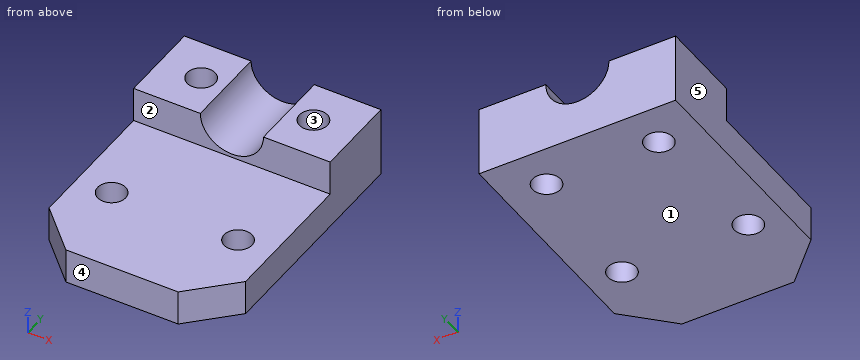
from build123d import *

# Parameters (mm, degrees)
SKETCH_1_R          = 2
EXTRUDE_1_DEPTH     = 10
CUT_EXTRUDE_2_REACH = 1024.045
SKETCH_2_W          = 6.505809731
SKETCH_2_H          = 33.357060804
SKETCH_3_R          = 4.5
CUT_EXTRUDE_3_DEPTH = 20


with BuildPart() as part:
    # 草图1 → 拉伸1 (new body)
    with BuildSketch(Plane.XY):
        Polygon((1243.510947309, 989.612625701), (1243.510947309, 1021.612625701), (1271.510947309, 1021.612625701), (1271.510947309, 989.612625701), (1265.510947309, 983.612625701), (1249.510947309, 983.612625701), align=None)
        with Locations((1265.510947309, 1015.612625701)):
            Circle(SKETCH_1_R, mode=Mode.SUBTRACT)
        with Locations((1249.510947309, 1015.612625701)):
            Circle(SKETCH_1_R, mode=Mode.SUBTRACT)
        with Locations((1248.510947309, 996.112625701)):
            Circle(SKETCH_1_R, mode=Mode.SUBTRACT)
        with Locations((1266.510947309, 996.112625701)):
            Circle(SKETCH_1_R, mode=Mode.SUBTRACT)
    extrude(amount=EXTRUDE_1_DEPTH)

    # 草图2 → 拉伸2 (cut, up to next)
    with BuildSketch(Plane.ZY.offset(-1243.510947309), mode=Mode.PRIVATE) as cut_extrude_2_sk1:
        with Locations((8.252904865, 992.934095299)):
            Rectangle(SKETCH_2_W, SKETCH_2_H)
    cut_extrude_2_tool1 = extrude(cut_extrude_2_sk1.sketch, amount=-CUT_EXTRUDE_2_REACH, mode=Mode.PRIVATE) & part.part
    add(cut_extrude_2_tool1.solids().sort_by_distance((1243.510947, 992.934095, 8.252905))[0], mode=Mode.SUBTRACT)

    # 草图3 → 拉伸3 (cut)
    with BuildSketch(Plane(origin=(0, 1021.612625701, 0), x_dir=(1, 0, 0), z_dir=(0, 1, 0))):
        with Locations((1257.510947309, -10)):
            Circle(SKETCH_3_R)
    extrude(amount=-CUT_EXTRUDE_3_DEPTH, mode=Mode.SUBTRACT)


solid = part.part
Design review of the part built by this model. Coordinates are the model's own, in mm. Face numbers are marked on the shaded views. A direction names the side the tool comes from. Coordinates: 2 decimals unless noted, no trailing zeros. Order: outer loops, then holes, each group sorted by start corner. A loop starts at its lowest first (then second) coordinate and runs counter-clockwise, first axis right, second up.
Item 1: Take a section at D-D, the plane y = 999. Write out the cut boundary in (x, z), then the cut area to 3 significant figures.
Item 2: For the marked faces 1 and 2, list the 3-axis set-ups (+Z, -Z, +X, -X, +Y, -Y) from which the entire face can be reached by the end or side of a thin tool; tool diameter is ignored.
Item 3: For pin 1 Ø8 at (x, y) = (1263.5, 1001.5) entering from +Z, flat-tipped, find the tip position at first contact; note if it passes through.
Item 4: The part is to be moulded in two halves that separate along X. For the marked faces 3, 4 and 5, say which applies: pulls with the +X half, pulls with the -X half, needs draft (parallel to the pull), parting line crosses it, or undercut.
Item 5: Take a section at A-A, the plane z = 7. Write out the cut boundary in (x, y), then the cut area to 3 significant figures.
Item 6: Take a section at C-C, the plane x = 1259. Write out the cut boundary in (y, z), then the cut area to 3 significant figures.
Item 7: For line 1 (Y direction, x = 1249, z = 2.25); line 2 (Y direction, x = 1249.75, z = 3.5); line 3 (X direction, y = 1016.5, z = 7.25), list the stretches that pass through material, from the lowest coordinate up.
Item 8: Take a section at B-B, the plane z = 1.25. Write out the cut boundary in (x, y), then the cut area to 3 significant figures.
The answers:
1. outline: (1243.51, 0) - (1271.51, 0) - (1271.51, 5) - (1243.51, 5) - close
1. area: 140 mm2
2. face 1: -Z, +X, -X, +Y, -Y
2. face 2: +Z, +X, -X, -Y
3. pin 1: stops at z = 5
4. face 3: undercut
4. face 4: needs draft
4. face 5: pulls with the -X half
5. outline: (1243.51, 1009.61) - (1254.16, 1009.61) - (1254.16, 1021.61) - (1243.51, 1021.61) - close; (1260.87, 1009.61) - (1271.51, 1009.61) - (1271.51, 1021.61) - (1260.87, 1021.61) - close; hole circle Ø4 at (1249.51, 1015.61); hole circle Ø4 at (1265.51, 1015.61)
5. area: 230 mm2
6. outline: (983.61, 0) - (1021.61, 0) - (1021.61, 5.75) - (1009.61, 5.75) - (1009.61, 5) - (983.61, 5) - close
6. area: 199 mm2
7. line 1: y = 984.12 to 994.17, 998.05 to 1013.68, 1017.55 to 1021.61
7. line 2: y = 983.61 to 994.54, 997.68 to 1013.63, 1017.6 to 1021.61
7. line 3: x = 1243.51 to 1247.72, 1251.3 to 1253.95, 1261.07 to 1263.72, 1267.3 to 1271.51
8. outline: (1243.51, 989.61) - (1249.51, 983.61) - (1265.51, 983.61) - (1271.51, 989.61) - (1271.51, 1021.61) - (1243.51, 1021.61) - close; hole circle Ø4 at (1248.51, 996.11); hole circle Ø4 at (1249.51, 1015.61); hole circle Ø4 at (1265.51, 1015.61); hole circle Ø4 at (1266.51, 996.11)
8. area: 978 mm2
